Study the drawing (mm; zero at the part's minimum x, y, z) and answer. A direction names the side the tool comes from. Coordinates: 2 decimals unless noted, no trailing zeros. Order: outer loops, then holes, each group sorted by start corner. A loop starts at its lowest first (then second) coordinate and runs counter-clockwise, first axis right, second up. Notation, with made-up numbers: (-11.5, 45.25) - (34.5, 45.25) arc R8 ccw to (34.5, 49.25) - close; hole circle Ø7 at (-38.5, 71.5). An arc over 180 degrees is marked (long way). Write item = value, one per line.
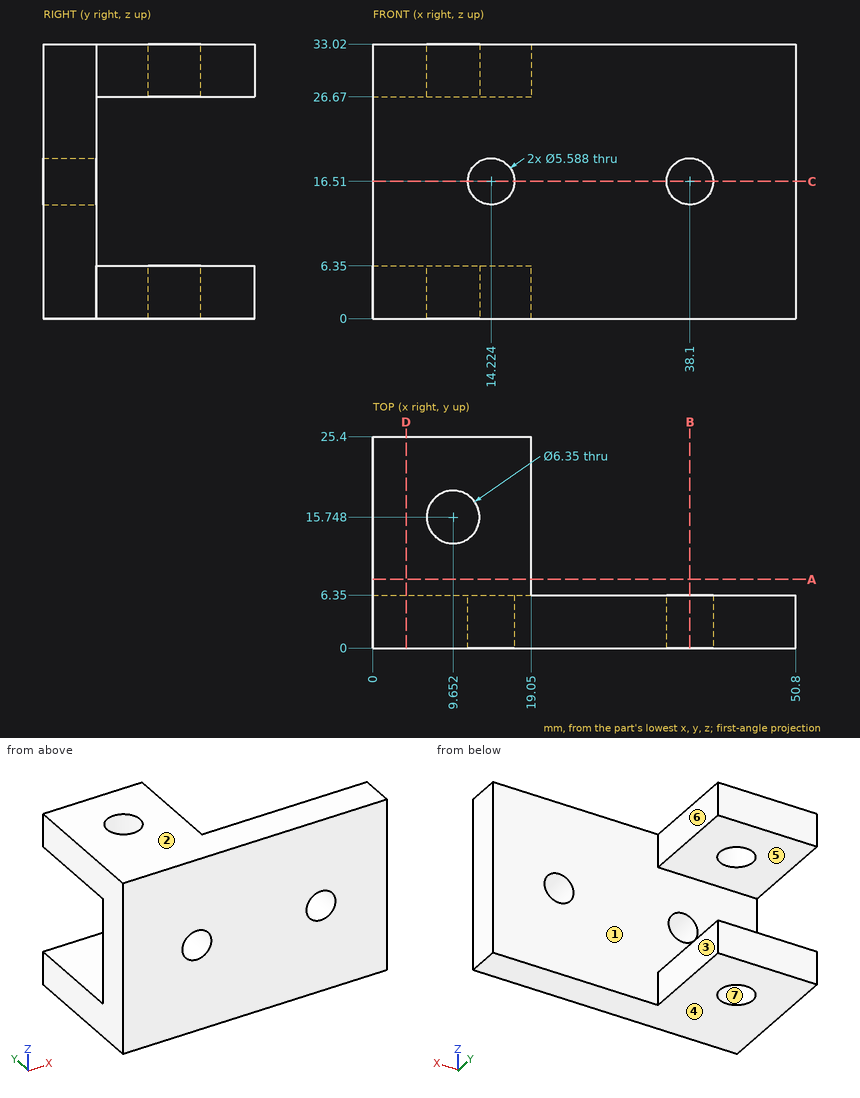
1) Determine the mould class of the marked faces 1, 2, 3 and 4 for opening direction Z: pulls with the +Z half, pulls with the -Z half, needs draft (parallel to the pull), parting line crosses it, or undercut.
Returned:
face_1 = undercut
face_2 = pulls with the +Z half
face_3 = needs draft
face_4 = pulls with the -Z half
2) The part is cut by section A-A (y = 8.25). Determine the outline of the cut face in (x, z), and give its area (3 significant figures).
Returned:
outline = (0, 0) - (19.05, 0) - (19.05, 6.35) - (0, 6.35) - close; (0, 26.67) - (19.05, 26.67) - (19.05, 33.02) - (0, 33.02) - close
area = 242 mm^2
3) The part is cut by section B-B (x = 38.1). Determine the outline of the cut face in (y, z).
Returned:
outline = (0, 0) - (6.35, 0) - (6.35, 13.72) - (0, 13.72) - close; (0, 19.3) - (6.35, 19.3) - (6.35, 33.02) - (0, 33.02) - close
4) For the marked faces 5, 6 and 7, determine the directions among +Z, -Z, +X, -X, +Y, -Y from which every point of the face is accessible in a straight line to the end or side of a thin tool.
Returned:
face_5 = +X, -X, +Y
face_6 = +Z, -Z, +X, +Y
face_7 = +Z, -Z
5) The part is cut by section D-D (x = 4). Determine the outline of the cut face in (y, z), and give its area (3 significant figures).
Returned:
outline = (0, 0) - (25.4, 0) - (25.4, 6.35) - (6.35, 6.35) - (6.35, 26.67) - (25.4, 26.67) - (25.4, 33.02) - (0, 33.02) - close
area = 452 mm^2
6) The part is cut by section C-C (z = 16.51). Determine the outline of the cut face in (x, y).
Returned:
outline = (0, 0) - (11.43, 0) - (11.43, 6.35) - (0, 6.35) - close; (17.02, 0) - (35.31, 0) - (35.31, 6.35) - (17.02, 6.35) - close; (40.89, 0) - (50.8, 0) - (50.8, 6.35) - (40.89, 6.35) - close
7) Flat-ended cylindrical pins translate along their axes: pin 1 Ø8 at (x, y) = (25.5, 12.5) entering from -Z; pin 2 Ø1.9 at (y, z) = (20, 2.5) entering from +X; pin 3 Ø5.5 at (x, y) = (5, 13) entering from -Z. Find the tip coordinate at first contact, or state that the pin passes through.
Returned:
pin_1 = through
pin_2 = 19.05
pin_3 = 0
8) Straight lines are drawn through the part: line 1 along Z through (x, y) = (2, 15.25); line 2 along X through (y, z) = (4, 14); line 3 along X through (y, z) = (2, 19). For each, find the intervals that lie inside material, in ascending order. Write a range as from..to.
Returned:
line_1 = 0..6.35, 26.67..33.02
line_2 = 0..13, 15.45..36.87, 39.33..50.8
line_3 = 0..12.96, 15.49..36.83, 39.37..50.8
